```python
from build123d import *

# Parameters (mm, degrees)
SKETCH1_R                  = 2.4638
BASE_FLANGE1_DEPTH         = 3.175
SKETCHED_START             = -25.4
SKETCHED_BEND1_DEPTH       = 70.78994652
SKETCHED_START_2           = 25.4
SKETCHED_BEND1_2_DEPTH     = 19.98994652
SKETCHED_START_3           = -10.2361999
SKETCHED_BEND1_3_DEPTH     = 20.4723998
SKETCHED_START_4           = -22.86
SKETCHED_BEND1_4_DEPTH     = 7.6961999
SKETCHED_START_5           = 15.1638001
SKETCHED_BEND1_5_DEPTH     = 7.6961999
SKETCHED_BEND1_6_DEPTH     = 70.78994652
SKETCHED_BEND1_7_DEPTH     = 50.8
SKETCHED_START_6           = -15.866732383
SKETCHED_BEND1_8_OUTLINE_R = 2.4638
SKETCHED_BEND1_8_DEPTH     = 3.866732383


with BuildPart() as part:
    # Base-Flange1: sheet metal written as solids
    # Sketch1 → Base-Flange1 (new body)
    with BuildSketch(Plane(origin=(0, 0, 0), x_dir=(1, 0, 0), z_dir=(0, 1, 0))):
        with BuildLine():
            Line((-35.2933, 25.4), (-132.557248776, -71.863948776))
            ThreePointArc((-132.557248776, -71.863948776), (-133.107851564, -74.632015918), (-130.761197552, -76.2))
            Line((-130.761197552, -76.2), (-66.10335348, -76.2))
            ThreePointArc((-66.10335348, -76.2), (-65.131337562, -76.006654013), (-64.307302256, -75.456051224))
            Line((-64.307302256, -75.456051224), (-36.037248776, -47.185997744))
            ThreePointArc((-36.037248776, -47.185997744), (-35.486645987, -46.361962438), (-35.2933, -45.38994652))
            Line((-35.2933, -45.38994652), (-15.5067, -45.38994652))
            Line((-15.5067, -45.38994652), (-15.5067, -25.4))
            Line((-15.5067, -25.4), (32.7533, -25.4))
            ThreePointArc((32.7533, -25.4), (34.549351224, -24.656051224), (35.2933, -22.86))
            Line((35.2933, -22.86), (35.2933, 22.86))
            ThreePointArc((35.2933, 22.86), (34.549351224, 24.656051224), (32.7533, 25.4))
            Line((32.7533, 25.4), (-35.2933, 25.4))
        make_face()
        with Locations(Location((-83.011763274, -58.239487758, 0), (0, 0, 270))):
            Circle(SKETCH1_R, mode=Mode.SUBTRACT)
        with Locations(Location((-65.051251031, -40.278975516, 0), (0, 0, 270))):
            Circle(SKETCH1_R, mode=Mode.SUBTRACT)
        with Locations(Location((9.8933, -12.7, 0), (0, 0, 270))):
            Circle(SKETCH1_R, mode=Mode.SUBTRACT)
        with Locations(Location((9.8933, 12.7, 0), (0, 0, 270))):
            Circle(SKETCH1_R, mode=Mode.SUBTRACT)
    extrude(amount=-BASE_FLANGE1_DEPTH)

    # Sketched Bend1: read off the stored shape, not the designer's step
    # Sketched Bend1 outline → Sketched Bend1 (cut)
    with BuildSketch(Plane.XY.offset(SKETCHED_START)):
        with BuildLine():
            Line((35.2933, 0), (-13.855493847, 0))
            ThreePointArc((-13.855493847, 0), (-15.205192704, -2.278520157), (-17.697112646, -3.175))
            Line((-17.697112646, -3.175), (35.2933, -3.175))
            Line((35.2933, -3.175), (35.2933, 0))
        make_face()
    extrude(amount=SKETCHED_BEND1_DEPTH, mode=Mode.SUBTRACT)

    # Sketched Bend1 2 outline → Sketched Bend1 2 (cut)
    with BuildSketch(Plane.XY.offset(SKETCHED_START_2)):
        Polygon((-15.5067, -0.854827941), (-15.5067, 0), (-16.683269724, 0), align=None)
    extrude(amount=SKETCHED_BEND1_2_DEPTH, mode=Mode.SUBTRACT)

    # Sketched Bend1 3 outline → Sketched Bend1 3 (add)
    with BuildSketch(Plane.XY.offset(SKETCHED_START_3)):
        with BuildLine():
            ThreePointArc((-13.855493847, 0), (-13.793115407, 0.98036242), (-13.976959977, 1.945350875))
            Line((-13.976959977, 1.945350875), (-28.998148559, 48.175815683))
            Line((-28.998148559, 48.175815683), (-32.017752998, 47.194686726))
            Line((-32.017752998, 47.194686726), (-16.996564416, 0.964221918))
            ThreePointArc((-16.996564416, 0.964221918), (-17.101190728, 0.303637383), (-17.697112646, 0))
            Line((-17.697112646, 0), (-13.855493847, 0))
        make_face()
    extrude(amount=SKETCHED_BEND1_3_DEPTH)

    # Sketched Bend1 4 outline → Sketched Bend1 4 (add)
    with BuildSketch(Plane.XY.offset(SKETCHED_START_4)):
        with BuildLine():
            ThreePointArc((-13.855493847, 0), (-13.793115407, 0.98036242), (-13.976959977, 1.945350875))
            Line((-13.976959977, 1.945350875), (-28.998148559, 48.175815683))
            Line((-28.998148559, 48.175815683), (-32.017752998, 47.194686726))
            Line((-32.017752998, 47.194686726), (-16.996564416, 0.964221918))
            ThreePointArc((-16.996564416, 0.964221918), (-17.101190728, 0.303637383), (-17.697112646, 0))
            Line((-17.697112646, 0), (-13.855493847, 0))
        make_face()
    extrude(amount=SKETCHED_BEND1_4_DEPTH)

    # Sketched Bend1 5 outline → Sketched Bend1 5 (add)
    with BuildSketch(Plane.XY.offset(SKETCHED_START_5)):
        with BuildLine():
            ThreePointArc((-13.855493847, 0), (-13.793115407, 0.98036242), (-13.976959977, 1.945350875))
            Line((-13.976959977, 1.945350875), (-28.998148559, 48.175815683))
            Line((-28.998148559, 48.175815683), (-32.017752998, 47.194686726))
            Line((-32.017752998, 47.194686726), (-16.996564416, 0.964221918))
            ThreePointArc((-16.996564416, 0.964221918), (-17.101190728, 0.303637383), (-17.697112646, 0))
            Line((-17.697112646, 0), (-13.855493847, 0))
        make_face()
    extrude(amount=SKETCHED_BEND1_5_DEPTH)

    # Sketched Bend1 6 outline → Sketched Bend1 6 (add)
    with BuildSketch(Plane.XY.offset(SKETCHED_START)):
        with BuildLine():
            ThreePointArc((-15.5067, -2.504188021), (-14.978553355, -2.0758811), (-14.532561771, -1.562580793))
            Line((-14.532561771, -1.562580793), (-15.5067, -0.854827941))
            Line((-15.5067, -0.854827941), (-15.5067, -2.504188021))
        make_face()
        with BuildLine():
            Line((-17.697112646, 0), (-16.683269724, 0))
            Line((-16.683269724, 0), (-17.101190728, 0.303637383))
            ThreePointArc((-17.101190728, 0.303637383), (-17.362703244, 0.080284594), (-17.697112646, 0))
        make_face()
    extrude(amount=SKETCHED_BEND1_6_DEPTH)

    # Sketched Bend1 7 outline → Sketched Bend1 7 (add)
    with BuildSketch(Plane.XY.offset(SKETCHED_START)):
        with BuildLine():
            ThreePointArc((-13.855493847, 0), (-13.793115407, 0.98036242), (-13.976959977, 1.945350875))
            Line((-13.976959977, 1.945350875), (-28.998148559, 48.175815683))
            Line((-28.998148559, 48.175815683), (-32.017752998, 47.194686726))
            Line((-32.017752998, 47.194686726), (-16.996564416, 0.964221918))
            ThreePointArc((-16.996564416, 0.964221918), (-16.969581414, 0.621370373), (-17.101190728, 0.303637383))
            Line((-17.101190728, 0.303637383), (-16.683269724, 0))
            Line((-16.683269724, 0), (-13.855493847, 0))
        make_face()
    extrude(amount=SKETCHED_BEND1_7_DEPTH)

    # Sketched Bend1 8 outline → Sketched Bend1 8 (cut)
    with BuildSketch(Plane(origin=(0, 0, 0), x_dir=(-0.30901699437495117, 0.9510565162951524, 0), z_dir=(0.9510565162951524, 0.3090169943749511, 0)).offset(SKETCHED_START_6)):
        with BuildLine():
            Line((54.778844143, -25.4), (54.778844143, -22.86))
            ThreePointArc((54.778844143, -22.86), (54.034895367, -24.656051224), (52.238844143, -25.4))
            Line((52.238844143, -25.4), (54.778844143, -25.4))
        make_face()
        with BuildLine():
            ThreePointArc((52.238844143, 25.4), (54.034895367, 24.656051224), (54.778844143, 22.86))
            Line((54.778844143, 22.86), (54.778844143, 25.4))
            Line((54.778844143, 25.4), (52.238844143, 25.4))
        make_face()
        with Locations((29.378844143, 12.7)):
            Circle(SKETCHED_BEND1_8_OUTLINE_R)
        with Locations((29.378844143, -12.7)):
            Circle(SKETCHED_BEND1_8_OUTLINE_R)
    extrude(amount=SKETCHED_BEND1_8_DEPTH, mode=Mode.SUBTRACT)


solid = part.part
```
Verification items for the finished model (mm, model axes). A direction names the side the tool comes from. Give positions to 0.01 mm unless a question says otherwise; leave off trailing zeros. Loops run counter-clockwise (first coordinate to the right, second up) from the corner with the lowest first, then second, coordinate; pieces in that order, holes last.
1. Section check A-A, the plane z = 17. Enter the section's corners in (x, y) (1 decimal).
2. Mould release check, pull along Y, two halves, no side actions. Record for faces 1 (the flat face through (-30.49, 47.69, -0.32)), 2 (the cylindrical face through (-23.406, 25.757, -11.96)), 3 (the cylindrical face through (-133.124, -1.565, 74.593)): released by +Y, released by -Y, zero draft, split by the parting line, or undercut.
3. Section check B-B, the plane x = -33.5. Enter the section's corners in (y, z) (3 decimals), then the cut area to 3 significant figures.
4. Thickness scan on line 1 (Y direction, x = -36, z = -20.5) (3 decimals); line 2 (X direction, y = 27.5, z = -12.5); line 3 (X direction, y = 46, z = -14). Record the ranges inside material, lowest first.
5. Set-up check for faces 4 (the flat face through (-83.244, -1.565, 22.551)), 5 (the flat face through (-25, -2, 45.39)), 6 (the flat face through (-24.61, 24.4, -0.36)): record each of +Z, -Z, +X, -X, +Y, -Y from which the full face is reachable in a straight line by a thin tool's end or side.
6. Section check C-C, the plane y = 30.5. Enter the section's corners in (x, z).
7. Go/stop test with flat-tipped pins: pin 1 Ø2 at (y, z) = (32.5, 15.5) entering from +X; pin 2 Ø4 at (x, z) = (-65.05, 40.28) entering from -Y; pin 3 Ø8.5 at (x, y) = (-20.5, 21.5) entering from +Z; pin 4 Ø8 at (x, z) = (-41.5, 23.5) entering from +Y. Record where each tip stops, or that it passes through.
Geometry says:
1. outline: (-77.7, -3.2) - (-17.7, -3.2) arc R3.9 ccw to (-14, 1.9) - (-29, 48.2) - (-32, 47.2) - (-17, 1) arc R0.7 cw to (-17.7, 0) - (-77.7, 0) - close
2. face 1: released by +Y
2. face 2: undercut
2. face 3: zero draft
3. outline: (-3.175, -25.4) - (0, -25.4) - (0, 45.39) - (-3.175, 45.39) - close
3. area: 225 mm2
4. line 1: y = -3.175 to 0
4. line 2: x = -25.62 to -22.28
4. line 3: x = -31.63 to -28.29
5. face 4: -Z, -X, +Y, -Y
5. face 5: +Z, +X, +Y, -Y
5. face 6: +Z, -Z, -X
6. outline: (-26.59, -25.4) - (-23.25, -25.4) - (-23.25, 25.4) - (-26.59, 25.4) - close
7. pin 1: stops at x = -23.58
7. pin 2: passes through
7. pin 3: stops at z = 25.4
7. pin 4: stops at y = 0
